```python
from build123d import *

# Parameters (mm, degrees)
SKETCH2_R               = 29.75
CUT_EXTRUDE2_DEPTH      = 21
CUT_EXTRUDE2_DEPTH_BACK = 21


with BuildPart() as part:
    # Sketch1 → Revolve1 (revolve)
    with BuildSketch(Plane(origin=(0, 0, 0), x_dir=(-1, 0, 0), z_dir=(0, 0, -1))):
        with BuildLine():
            Line((-12.7, 4.956029105), (-18.888228568, 3.297898257))
            ThreePointArc((-18.888228568, 3.297898257), (-19.69003001, 2.762151662), (-20, 1.849009518))
            Line((-20, 1.849009518), (-20, 0))
            Line((-20, 0), (-11.85, 0))
            Line((-11.85, 0), (-11.85, 2.5))
            Line((-11.85, 2.5), (-11.05, 2.5))
            Line((-11.05, 2.5), (-11.05, 70))
            Line((-11.05, 70), (-12.7, 70))
            Line((-12.7, 70), (-12.7, 4.956029105))
        make_face()
    revolve(axis=Axis((0, 0, 0), (0, 1, 0)))

    # Sketch2 → Cut-Extrude2 (cut, two sides)
    with BuildSketch(Plane(origin=(0, 0, 0), x_dir=(0, 0, -1), z_dir=(1, 0, 0))) as cut_extrude2_sk:
        with Locations((0, 84.706029105)):
            Circle(SKETCH2_R)
    extrude(amount=CUT_EXTRUDE2_DEPTH, mode=Mode.SUBTRACT)
    extrude(cut_extrude2_sk.sketch, amount=-CUT_EXTRUDE2_DEPTH_BACK, mode=Mode.SUBTRACT)


solid = part.part
```
For this review, take the finished solid that the model builds, in its own axes (mm). A direction names the side the tool comes from. Give positions to 0.01 mm unless a question says otherwise; leave off trailing zeros. Write each loop counter-clockwise with the first axis right and the second up, starting at its lowest first coordinate (ties: lowest second). Pieces come first, ordered by that corner, then holes.
Item 1: Take a section at B-B (z = 0). Give the boundary of the cut face in (x, y), and give its area (3 significant figures).
Item 2: Take a section at A-A (x = 0). Give the boundary of the cut face in (y, z), and give its area (3 significant figures).
Item 3: The part is to be moulded in two halves that separate along Z. For faces 3 (the face through (8, 2.5, 8)), 4 (the face through (-2.395, 30.175, 10.787)), 5 (the face through (-4.336, 0.912, 19.524)), 6 (the face through (9, 0, 9)), say which applies: +Z half, -Z half, draft (parallel to the pull), parting line (faces both ways), or undercut.
Item 4: Wall thickness on probe 1 along X at (y, z) = (42.5, 0); probe 2 along X at (y, z) = (1, 0): over which ranges is each line inside the solid? List them lowest first.
Item 5: Take a section at C-C (y = 46.5). Give the boundary of the cut face in (x, z).
Item 6: Insertion check: P1, Ø3, axis at x = 9.5, y = 46, coming from the -Z side; P2, Ø6, axis at x = 10, y = 51, coming from the -Z side; P3, Ø19, axis at x = 0, z = 0, coming from the -Y side; P4, Ø5, axis at y = 48, z = 11.5, coming from the +X side. Each pin has a flat end and moves straight along its axis. Give the tip position at first contact, or say it passes through.
Item 7: Machinability: for faces 1 (the face through (-2.75, 31.01, 12.4)), 2 (the face through (11.303, 1.268, -3.559)), which of the approach directions +Z, -Z, +X, -X, +Y, -Y give a long, thin tool a straight path to every point of the face, cutting with its end or side? Answer none if there is none.
Established:
1. outline: (-20, 0) - (-11.85, 0) - (-11.85, 2.5) - (-11.05, 2.5) - (-11.05, 54.96) - (-12.7, 54.96) - (-12.7, 4.96) - (-18.89, 3.3) arc R1.5 ccw to (-20, 1.85) - close; (11.05, 2.5) - (11.85, 2.5) - (11.85, 0) - (20, 0) - (20, 1.85) arc R1.5 ccw to (18.89, 3.3) - (12.7, 4.96) - (12.7, 54.96) - (11.05, 54.96) - close
1. area: 235 mm2
2. outline: (0, -20) - (1.85, -20) arc R1.5 ccw to (3.3, -18.89) - (4.96, -12.7) - (57.8, -12.7) arc R29.75 cw to (57.08, -11.05) - (2.5, -11.05) - (2.5, -11.85) - (0, -11.85) - close; (0, 11.85) - (2.5, 11.85) - (2.5, 11.05) - (57.08, 11.05) arc R29.75 cw to (57.8, 12.7) - (4.96, 12.7) - (3.3, 18.89) arc R1.5 ccw to (1.85, 20) - (0, 20) - close
2. area: 243 mm2
3. face 3: undercut
3. face 4: undercut
3. face 5: parting line
3. face 6: draft
4. probe 1: x = -12.7 to -11.05, 11.05 to 12.7
4. probe 2: x = -20 to -11.85, 11.85 to 20
5. outline: circle Ø25.4 at (0, 0); hole circle Ø22.1 at (0, 0)
6. P1: stops at z = -9.86
6. P2: stops at z = -10.6
6. P3: passes through
6. P4: stops at x = 8.96
7. face 1: +Y
7. face 2: -Y
